Part model, mm, in its own coordinate system. A direction names the side the tool comes from. Give positions to 0.01 mm unless a question says otherwise; leave off trailing zeros. Write each loop counter-clockwise with the first axis right and the second up, starting at its lowest first coordinate (ties: lowest second). Pieces come first, ordered by that corner, then holes.
Autodesk Inventor part; units mm, degrees
ref_plane "Work Plane4" through (-34.8055, 8.3289, 16.6138) normal (0.7071068, -0.7071068, 0) x (0.7071068, 0.7071068, 0)
ref_plane "Work Plane5" through (-45.7299, 3.9099, 44.1) normal (0, 0, -1) x (0, 1, 0)
ref_plane "YZ Plane" through (0, 0, 0) normal (1, 0, 0) x (0, 1, 0)
ref_plane "Work Plane1" through (0, 0, 10) normal (0, 0, 1) x (1, 0, 0)
sketch "Sketch1" plane through (0, 0, 10) normal (0, 0, 1) x (1, 0, 0)
  line L0 (-4.0299, -0.3538) -> (-2.2322, 1.4439) construction
  arc A0 (-1.4439, 2.2322) -> (-2.2322, 1.4439) centre (-0.9299, 0.9299) ccw construction
  line L1 (-1.4439, 2.2322) -> (0.3538, 4.0299) construction
  line L2 (-37.8299, 42.8299) -> (-37.8299, 37.8299) construction
  line L3 (-37.8299, 37.8299) -> (-42.9208, 37.8299) construction
  line L4 (-37.8299, 42.2137) -> (-37.8299, 45.8299) construction
  line L5 (-37.8299, 45.8299) -> (-4.0299, 45.8299) construction
  line L6 (-4.0299, 45.8299) -> (-4.0299, 42.2137) construction
  line L7 (-4.0299, 4.0299) -> (0.3538, 4.0299)
  circle A1 centre (-20.9299, 20.9299) radius 17.5
  line L8 (-20.9299, 58.9723) -> (17.1124, 20.9299) construction
  line L9 (17.1124, 20.9299) -> (-20.9299, -17.1124) construction
  line L10 (-20.9299, -17.1124) -> (-58.9723, 20.9299) construction
  line L11 (-58.9723, 20.9299) -> (-20.9299, 58.9723) construction
  line L12 (-20.9299, 58.9723) -> (-20.9299, -17.1124) construction
  line L13 (17.1124, 20.9299) -> (-58.9723, 20.9299) construction
  line L14 (-20.9299, 58.9723) -> (32.8701, 58.9723) construction
  line L15 (-43.4299, 43.4299) -> (1.5701, 43.4299) construction
  line L16 (1.5701, 43.4299) -> (1.5701, -1.5701) construction
  line L17 (1.5701, -1.5701) -> (-43.4299, -1.5701) construction
  line L18 (-43.4299, -1.5701) -> (-43.4299, 43.4299) construction
  line L19 (-43.4299, 43.4299) -> (1.5701, -1.5701) construction
  line L20 (1.5701, 43.4299) -> (-43.4299, -1.5701) construction
  line L21 (-43.4299, 5.3876) -> (-43.4299, 36.4723)
  line L22 (-43.4299, 36.4723) -> (-36.4723, 43.4299)
  line L23 (-36.4723, 43.4299) -> (-5.3876, 43.4299)
  line L24 (-5.3876, 43.4299) -> (1.5701, 36.4723)
  line L25 (1.5701, 36.4723) -> (1.5701, 5.3876)
  line L26 (1.5701, 5.3876) -> (-5.3876, -1.5701)
  line L27 (-5.3876, -1.5701) -> (-36.4723, -1.5701)
  line L28 (-36.4723, -1.5701) -> (-43.4299, 5.3876)
  line L29 (-4.0299, 42.2137) -> (-37.8299, 42.2137)
  line L30 (-4.0299, -0.3538) -> (-4.0299, 4.0299)
  circle A2 centre (-20.9299, 20.9299) radius 1.4
  line L31 (-10.9299, 10.9299) -> (-30.9299, 10.9299) construction
  line L32 (-30.9299, 10.9299) -> (-30.9299, 30.9299) construction
  line L33 (-30.9299, 30.9299) -> (-10.9299, 30.9299) construction
  line L34 (-10.9299, 30.9299) -> (-10.9299, 10.9299) construction
  line L35 (-10.9299, 10.9299) -> (-30.9299, 30.9299) construction
  line L36 (-30.9299, 10.9299) -> (-10.9299, 30.9299) construction
  circle A3 centre (-30.9299, 30.9299) radius 1.4
  circle A4 centre (-30.9299, 10.9299) radius 1.4
  circle A5 centre (-10.9299, 10.9299) radius 1.4
  line L37 (-45.8299, 37.8299) -> (-42.0723, 37.8299) construction
  line L38 (-42.1723, 37.7299) -> (-45.8299, 37.7299)
  line L39 (-45.8299, 37.7299) -> (-45.8299, 4.1299)
  line L40 (-45.8299, 4.1299) -> (-42.1723, 4.1299)
  line L41 (-42.1723, 4.1299) -> (-42.1723, 37.7299)
  line L42 (-45.8299, 4.0299) -> (-42.0723, 4.0299) construction
  line L43 (-45.8299, 37.8299) -> (-42.0723, 37.8299)
  line L44 (-37.7299, 45.8299) -> (-4.1299, 45.8299)
  line L45 (-4.1299, 45.8299) -> (-4.1299, 42.1723)
  line L46 (-4.1299, 42.1723) -> (-37.7299, 42.1723)
  line L47 (-37.7299, 42.1723) -> (-37.7299, 45.8299)
  line L48 (0.4701, 37.8299) -> (0.4701, 4.0299) construction
  line L49 (0.4701, 4.0299) -> (3.9701, 4.0299) construction
  line L50 (3.9701, 37.8299) -> (3.9701, 4.0299) construction
  line L51 (0.4701, 37.8299) -> (3.9701, 37.8299) construction
  line L52 (-45.8299, -3.9701) -> (-4.0299, -3.9701) construction
  line L53 (0.3124, 37.7299) -> (3.9701, 37.7299)
  line L54 (3.9701, 37.7299) -> (3.9701, 4.1299)
  line L55 (3.9701, 4.1299) -> (0.3124, 4.1299)
  line L56 (0.3124, 4.1299) -> (0.3124, 37.7299)
  line L57 (-4.1713, -0.3538) -> (-37.7299, -0.3538)
  line L58 (-37.7299, -0.3538) -> (-37.7299, -3.9701)
  line L59 (-37.7299, -3.9701) -> (-4.1713, -3.9701)
  line L60 (-4.1713, -3.9701) -> (-4.1713, -0.3538)
  point P0 (-37.8299, 4.0299)
  dimension "d18" = 53.8
  dimension "d19" = 45
  dimension "d20" = 53.8
  dimension "d21" = 45
  dimension "d22" = 45
  dimension "d30" = 20
  dimension "d31" = 20
  dimension "d32" = 2.8
  dimension "d33" = 2.8
  dimension "d34" = 2.8
  dimension "d35" = 2.8
  dimension "d36" = 0.1
  dimension "d37" = 0.1
  dimension "d38" = 0.1
  dimension "d39" = 0.1
extrude "Extrusion1" add sketch "Sketch1" along normal blind 5 contours L30 L26 L57 L28 L41 L22 L46 L24 L56 L7 | L7 L26 L30 | L56 L24 L25 L26 | L26 L25 L24 L53 L54 L55 | L60 L59 L58 L57 L28 L27 L26 | L26 L27 L28 L57 | L46 L22 L29 L24 | L24 L29 L45 | L40 L39 L38 L22 L21 L28 | L28 L21 L22 L41 | L29 L22 L23 L24 | L24 L23 L22 L29 L47 L44 L45 | L47 L29 L22 | A1 | A2 | A3 | A4 | A5
sketch "Sketch4" plane through (0, 0, 15) normal (0, 0, 1) x (1, 0, 0)
  line L0 (-37.7299, 42.1723) -> (-42.1723, 37.7299)
  line L1 (-42.1723, 37.7299) -> (-45.8299, 37.7299)
  line L2 (-45.8299, 37.7299) -> (-45.8299, 4.1299)
  line L3 (-45.8299, 4.1299) -> (-42.1723, 4.1299)
  line L4 (-42.1723, 4.1299) -> (-37.6885, -0.3538)
  line L5 (-37.6885, -0.3538) -> (-37.7299, -0.3538)
  line L6 (-37.7299, -0.3538) -> (-37.7299, -3.9701)
  line L7 (-37.7299, -3.9701) -> (-4.1713, -3.9701)
  line L8 (-4.1713, -3.9701) -> (-4.1713, -0.3538)
  line L9 (-4.1713, -0.3538) -> (0.3124, 4.1299)
  line L10 (0.3124, 4.1299) -> (3.9701, 4.1299)
  line L11 (3.9701, 4.1299) -> (3.9701, 37.7299)
  line L12 (3.9701, 37.7299) -> (0.3124, 37.7299)
  line L13 (0.3124, 37.7299) -> (-4.1299, 42.1723)
  line L14 (-4.1299, 42.1723) -> (-4.1299, 45.8299)
  line L15 (-4.1299, 45.8299) -> (-37.7299, 45.8299)
  line L16 (-37.7299, 45.8299) -> (-37.7299, 42.1723)
  line L17 (-45.8299, 37.7299) -> (-45.8299, 4.1299)
  line L18 (-45.8299, 7.911) -> (-7.911, 45.8299)
  line L19 (-45.8299, 7.911) -> (7.7955, 7.911) construction
  line L20 (-7.911, 45.8299) -> (-19.2247, 45.8299)
  line L21 (-4.1299, 45.8299) -> (-37.7299, 45.8299)
  line L22 (-19.2247, 45.8299) -> (-45.8299, 19.2247)
  line L23 (-45.8299, 7.911) -> (-45.8299, 19.2247)
  circle A0 centre (-40.9299, 0.9299) radius 1.1933
  circle A1 centre (-0.9299, 40.9299) radius 1.4
  line L24 (-40.9299, 0.9299) -> (-0.9299, 40.9299)
  line L25 (0.3124, 37.7299) -> (-4.1299, 42.1723)
  point P0 (0, 0)
  dimension "d40" = 45
  dimension "d41" = 8
extrude "Extrusion4" add sketch "Sketch4" along normal blind 28 contours L15 L18 L2 L22
sketch "Sketch5" plane through (-45.8299, 19.2247, 15) normal (-0.7071068, 0.7071068, 0) x (-0.7071068, -0.7071068, 0)
  line L0 (0, 0) -> (-37.6254, 0)
  line L1 (0, 0) -> (0, 28)
  line L2 (-37.6254, 28) -> (0, 28)
  line L3 (-37.6254, 0) -> (-37.6254, 28)
  circle A0 centre (-18.8127, 9.1873) radius 18.8127
  line L4 (-6.8127, 24) -> (-36.8127, 24) construction
  line L5 (-36.8127, 24) -> (-36.8127, 4) construction
  line L6 (-36.8127, 4) -> (-6.8127, 4) construction
  line L7 (-6.8127, 4) -> (-6.8127, 24) construction
  line L8 (-6.8127, 24) -> (-36.8127, 4) construction
  line L9 (-36.8127, 24) -> (-6.8127, 4) construction
  point P0 (-18.8127, -15)
  point P1 (-21.8127, 14)
  dimension "d44" = 30
  dimension "d45" = 20
hole "Hole1" at (-19.7994, 45.2552, 39) at (-19.7994, 45.2552, 19) at (-41.0126, 24.042, 39) at (-30.406, 34.6486, 29) direction (0.7071068, -0.7071068, 0) diameter 2.9 depth 12
sketch "Sketch6" plane through (-37.7299, -3.9701, 10) normal (0, -1, 0) x (1, 0, 0)
  circle A0 centre (-3.2, 36.9) radius 1.45
  circle A1 centre (36.8, 36.9) radius 1.45
  line L0 (-6.1, 0) -> (-6.1, 39.8)
  line L1 (-0.1, 0) -> (-6.1, 0)
  line L2 (-0.1, 33.8) -> (-0.1, 0)
  line L3 (33.7, 33.8) -> (-0.1, 33.8)
  line L4 (33.7, 33.8) -> (33.7, 0)
  line L5 (39.7, 0) -> (33.7, 0)
  line L6 (39.7, 39.8) -> (39.7, 0)
  line L7 (-6.1, 39.8) -> (39.7, 39.8)
  circle A2 centre (16.8, 16.9) radius 16.9
  circle A3 centre (16.8, 16.9) radius 14.9
  line L8 (-0.1, 16.9) -> (-0.1, 0)
  line L9 (0, 0) -> (33.5586, 0)
  line L10 (0.0414, 0) -> (-4.4423, 0)
  line L11 (33.5586, 0) -> (0.0414, 0)
  line L12 (33.7, 16.9) -> (33.5586, 0)
  point P0 (37.7299, -10)
  dimension "d53" = 2
extrude "Extrusion5" cut sketch "Sketch6" against normal up to surface contours A3 surface through (-45.8299, 7.911, 15) normal (0.7071068, -0.7071068, 0)
ref_plane "Work Plane3" through (3.9701, 45.8299, 26) normal (1, 0, 0) x (0, -1, 0)
sketch "Sketch7" plane through (3.9701, 45.8299, 26) normal (1, 0, 0) x (0, -1, 0)
  line L0 (41.8, -17.8) -> (41.8, 16)
  line L1 (8, -17.8) -> (41.8, -17.8)
  line L2 (8, -17.8) -> (8, 16)
  circle A0 centre (24.9, -0.9) radius 16.9
  circle A1 centre (24.9, -0.9) radius 14.9
  point P0 (45.8299, 26)
  dimension "d56" = 2
ref_plane "Work Plane4" through (-34.8055, 8.3289, 16.6138) normal (0.7071068, -0.7071068, 0) x (0.7071068, 0.7071068, 0)
extrude "Extrusion6" cut sketch "Sketch7" against normal up to surface contours A1 surface through (-45.8299, 7.911, 15) normal (0.7071068, -0.7071068, 0)
sketch "Sketch8" plane through (-45.8299, 19.2247, 15) normal (-0.7071068, 0.7071068, 0) x (-0.7071068, -0.7071068, 0)
  arc A0 (-37.6254, 2.7992) -> (-37.6254, 5.2008) centre (-36.8127, 4) ccw
  circle A1 centre (-36.8127, 4) radius 7.5
  point P0 (-18.8127, -15)
  dimension "d59" = 15
extrude "Extrusion7" cut sketch "Sketch8" along normal blind 10
sketch "Sketch9" plane through (0, 0, 10) normal (0, 0, -1) x (-1, 0, 0)
  line L0 (45.8299, 19.2247) -> (24.2855, 40.7692)
  line L1 (41.7776, 11.9633) -> (26.8705, 26.8705)
  line L2 (26.8705, 26.8705) -> (11.9633, 41.7776)
  line L3 (19.2247, 45.8299) -> (24.2855, 40.7692)
  line L4 (7.911, 45.8299) -> (11.9633, 41.7776)
  line L5 (41.7776, 11.9633) -> (45.8299, 7.911)
  line L6 (15.1679, 38.5731) -> (20.8247, 44.2299)
  line L7 (13.1172, 40.6237) -> (18.3235, 45.8299)
  line L8 (34.3304, 19.4105) -> (39.9873, 25.0673)
  line L9 (36.3811, 17.3599) -> (42.0379, 23.0167)
  circle A0 centre (20.5065, 38.8913) radius 1.4
  line L10 (25.7745, 27.9665) -> (31.4313, 33.6233)
  line L11 (31.4313, 33.6233) -> (25.7745, 27.9665)
  line L12 (26.8705, 26.8705) -> (32.5273, 32.5273)
  circle A1 centre (38.8913, 20.5065) radius 1.4
  point P0 (0, 0)
  point P1 (34.7528, 24.7491)
  dimension "d62" = 2.8
hole "Hole2" at (-20.5065, 38.8913, 10) at (-38.8913, 20.5065, 10) direction (0, 0, 1) diameter 2.8 depth 12 counterbore diameter 5.5 counterbore depth 3
sketch "Sketch11" plane through (0, 0, 43) normal (0, 0, 1) x (1, 0, 0)
  line L0 (-7.911, 45.8299) -> (-19.2247, 45.8299)
  line L1 (-19.2247, 45.8299) -> (-45.8299, 19.2247)
  line L2 (-45.8299, 19.2247) -> (-45.8299, 7.911)
  line L3 (-45.8299, 7.911) -> (-7.911, 45.8299)
  line L4 (-45.8299, 37.7299) -> (-45.8299, 19.2247)
  line L5 (-42.1723, 37.7299) -> (-45.8299, 37.7299)
  line L6 (-37.7299, 42.1723) -> (-42.1723, 37.7299)
  line L7 (-37.7299, 45.8299) -> (-37.7299, 42.1723)
  line L8 (-29.3463, 45.8299) -> (-37.7299, 45.8299)
  line L9 (-29.3463, 45.8299) -> (-19.2247, 45.8299)
  line L10 (-4.1299, 45.8299) -> (-7.911, 45.8299)
  line L11 (-4.1299, 42.1723) -> (-4.1299, 45.8299)
  line L12 (0.3124, 37.7299) -> (-4.1299, 42.1723)
  line L13 (3.9701, 37.7299) -> (0.3124, 37.7299)
  line L14 (3.9701, 29.8965) -> (3.9701, 11.9633)
  line L15 (3.9701, 29.8965) -> (3.9701, 37.7299)
  line L16 (-11.9633, -3.9701) -> (-4.1713, -3.9701)
  line L17 (-4.1713, -3.9701) -> (-4.1713, -0.3538)
  line L18 (-4.1713, -0.3538) -> (0.3124, 4.1299)
  line L19 (0.3124, 4.1299) -> (3.9701, 4.1299)
  line L20 (3.9701, 4.1299) -> (3.9701, 11.9633)
  line L21 (-11.9633, -3.9701) -> (-29.8965, -3.9701)
  line L22 (-37.7299, -3.9701) -> (-29.8965, -3.9701)
  line L23 (-37.7299, -0.3538) -> (-37.7299, -3.9701)
  line L24 (-45.8299, 7.911) -> (-7.911, 45.8299)
  line L25 (-45.8299, 7.911) -> (-7.911, 45.8299)
  line L26 (-45.8299, 7.911) -> (-45.8299, 4.1299)
  line L27 (-45.8299, 4.1299) -> (-42.1723, 4.1299)
  line L28 (-37.6885, -0.3538) -> (-37.7299, -0.3538)
  line L29 (-42.1723, 4.1299) -> (-37.6885, -0.3538)
  point P0 (0, 0)
extrude "Extrusion8" cut sketch "Sketch11" against normal through all contours L10 L11 L12 L13 L15 L14 L20 L19 L18 L17 L16 L21 L22 L23 L28 L29 L27 L26 L3 | L1 L4 L5 L6 L7 L8 L9
sketch "Sketch12" plane through (-45.8299, 19.2247, 10) normal (-0.7071068, 0.7071068, 0) x (-0.7071068, -0.7071068, 0)
  line L0 (-45.6254, 33) -> (-45.6254, 0)
  line L1 (8, 0) -> (8, 33)
  line L2 (-45.6254, 0) -> (8, 0)
  line L3 (8, 0) -> (8, 4)
  line L4 (8, 4) -> (-45.6254, 4)
  line L5 (-45.6254, 4) -> (-45.6254, 0)
  point P0 (-18.8127, -10)
  point P1 (45.6254, -4)
  point P2 (45.6254, -5)
  point P3 (-8, -5)
  point P4 (-8, -4)
  dimension "d73" = 4
extrude "Extrusion9" cut sketch "Sketch12" against normal blind 29
sketch "Sketch13" plane through (0, 0, 43) normal (0, 0, 1) x (1, 0, 0)
  line L0 (-7.911, 45.8299) -> (-19.2247, 45.8299)
  line L1 (-19.2247, 45.8299) -> (-45.8299, 19.2247)
  line L2 (-45.8299, 19.2247) -> (-45.8299, 7.911)
  line L3 (-45.8299, 7.911) -> (-7.911, 45.8299)
  point P0 (0, 0)
ref_plane "Work Plane5" through (-45.7299, 3.9099, 44.1) normal (0, 0, -1) x (0, 1, 0)
extrude "Extrusion10" add sketch "Sketch13" along normal up to surface (1.1 mm away)
properties part number "20_Cube_Insert_Kinematic_Mirrormount_45_base_part2"
1) Saw through at A-A (z = 18.5). State how many separate pieces and enclosed holes the cut face has, and give its area (3 significant figures).
Check result:
separate pieces: 2
enclosed holes: 2
area: 331 mm2
2) Mould opens along Y. For faces 1 (the cylindrical face through (-17.948, 41.371, 38.811)), 2 (the flat face through (-27.136, 26.605, 28.839)), 3 (the flat face through (-45.83, 14, 29)), 4 (the flat face through (-32.341, 32.714, 28.839)) say: +Y half, -Y half, draft (parallel to the pull), parting line (faces both ways), or undercut.
Check result:
face 1: undercut
face 2: -Y half
face 3: draft
face 4: +Y half
3) Saw through at D-D (y = 26.5). Write the cut outline in (x, z), and give its area (3 significant figures).
Check result:
outline: (-38.55, 14) - (-27.24, 14) - (-27.24, 44.1) - (-38.55, 44.1) - close
area: 341 mm2
4) Flat gauge pins, fed straight in: P1, Ø6, axis at y = 35, z = 18, coming from the -X side; P2, Ø1.5, axis at y = 27, z = 35, coming from the -X side; P3, Ø8, axis at x = -13, z = 22.5, coming from the -Y side. Where does each tip first touch, or does it go through?
Check result:
P1: stops at x = -33.05
P2: stops at x = -38.8
P3: stops at y = 36.74
5) Saw through at C-C (z = 42.5). Write the cut outline in (x, y), and give its area (3 significant figures).
Check result:
outline: (-45.83, 7.91) - (-7.91, 45.83) - (-19.22, 45.83) - (-45.83, 19.22) - close
area: 365 mm2
6) Drill centre lines: L1, parallel to Y at x = -19.5, z = 24; L2, parallel to Y at x = -17, z = 40; L3, parallel to Y at x = -21, z = 24. Where is each one in solid material? Low to high.
Check result:
L1: y = 34.24 to 45.55
L2: y = 36.74 to 40.97, 43.94 to 45.83
L3: y = 32.74 to 44.05
7) 3-axis set-ups, long thin cutter, end or side, ignore diameter. For faces 5 (the flat face through (-21, 39, 22)), 6 (the flat face through (-30, 30, 44.1)): which of +Z, -Z, +X, -X, +Y, -Y reach the whole face in a straight line?
Check result:
face 5: -Z
face 6: +Z, +X, -X, +Y, -Y
